Geometry: final body of the model. Coordinates: model frame, mm. Face numbers are marked on the shaded views. A direction names the side the tool comes from. Give positions to 0.01 mm unless a question says otherwise; leave off trailing zeros. Loops run counter-clockwise (first coordinate to the right, second up) from the corner with the lowest first, then second, coordinate; pieces in that order, holes last.
Autodesk Inventor part; units mm, degrees
ref_plane "YZ Plane" through (0, 0, 0) normal (1, 0, 0) x (0, 1, 0)
ref_plane "XZ Plane" through (0, 0, 0) normal (0, 1, 0) x (-1, 0, 0)
ref_plane "XY Plane" through (0, 0, 0) normal (0, 0, 1) x (1, 0, 0)
sketch "Sketch1" plane through (0, 0, 0) normal (0, 0, 1) x (1, 0, 0)
  line L0 (-24.5, 22.5) -> (24.5, 22.5)
  line L1 (29.5, 17.5) -> (29.5, -17.5)
  line L2 (24.5, -22.5) -> (-24.5, -22.5)
  line L3 (-29.5, -17.5) -> (-29.5, 17.5)
  arc A0 (-24.5, 22.5) -> (-29.5, 17.5) centre (-24.5, 17.5) ccw
  arc A1 (29.5, 17.5) -> (24.5, 22.5) centre (24.5, 17.5) ccw
  arc A2 (24.5, -22.5) -> (29.5, -17.5) centre (24.5, -17.5) ccw
  arc A3 (-29.5, -17.5) -> (-24.5, -22.5) centre (-24.5, -17.5) ccw
  line L4 (-24.5, 19.5) -> (24.5, 19.5)
  line L5 (24.5, -19.5) -> (-24.5, -19.5)
  arc A4 (-24.5, 19.5) -> (-26.5, 17.5) centre (-24.5, 17.5) ccw
  arc A5 (-26.5, -17.5) -> (-24.5, -19.5) centre (-24.5, -17.5) ccw
  arc A6 (26.5, 17.5) -> (24.5, 19.5) centre (24.5, 17.5) ccw
  arc A7 (24.5, -19.5) -> (26.5, -17.5) centre (24.5, -17.5) ccw
  line L6 (-26.5, -16.5) -> (-24.5, -16.5)
  line L7 (-24.5, -16.5) -> (-24.5, -14.5)
  line L8 (-24.5, -14.5) -> (-26.5, -14.5)
  line L9 (-26.5, -12.5) -> (-24.5, -12.5)
  line L10 (-24.5, -12.5) -> (-24.5, -10.5)
  line L11 (-24.5, -10.5) -> (-26.5, -10.5)
  line L12 (26.5, -16.5) -> (24.5, -16.5)
  line L13 (24.5, -14.5) -> (26.5, -14.5)
  line L14 (26.5, -12.5) -> (24.5, -12.5)
  line L15 (24.5, -10.5) -> (26.5, -10.5)
  line L16 (-26.5, -10.5) -> (-26.5, 17.5)
  line L17 (-26.5, -17.5) -> (-26.5, -16.5)
  line L18 (-26.5, -14.5) -> (-26.5, -12.5)
  line L19 (26.5, 17.5) -> (26.5, -10.5)
  line L20 (26.5, -12.5) -> (26.5, -14.5)
  line L21 (26.5, -16.5) -> (26.5, -17.5)
  line L22 (24.5, -12.5) -> (24.5, -10.5)
  line L23 (24.5, -16.5) -> (24.5, -14.5)
  point P0 (0, 0)
  point P1 (0, 22.5)
  point P2 (-29.5, 0)
  point P3 (0, 19.5)
  point P4 (-26.5, 0)
  dimension "d0" = 5
  dimension "d1" = 59
  dimension "d2" = 45
  dimension "d4" = 3
  dimension "d6" = 3
  dimension "d7" = 2
  dimension "d8" = 2
  dimension "d9" = 3
extrude "Extrusion1" add sketch "Sketch1" along normal blind 10
sketch "Sketch3" plane through (-29.5, -17.5, 0) normal (-1, 0, 0) x (0, 0, 1)
  line L0 (0, 0) -> (0, 35)
  line L1 (0, 0) -> (10, 0)
  line L2 (10, 35) -> (10, 0)
  line L3 (0, 35) -> (10, 35)
  line L4 (5, 31) -> (5, 4) construction
  point P0 (0, 17.5)
  point P1 (5, 35)
  point P2 (0, 17.5)
  point P3 (5, 17.5)
  dimension "d20" = 27
sketch "Sketch2" plane through (-24.5, 22.5, 0) normal (0, 1, 0) x (1, 0, 0)
  line L0 (0, 0) -> (49, 0)
  line L1 (0, 0) -> (0, -10)
  line L2 (49, -10) -> (0, -10)
  line L3 (49, 0) -> (49, -10)
  line L4 (7, -5) -> (42, -5) construction
  point P0 (24.5, 0)
  point P1 (0, -5)
  point P2 (24.5, 0)
  point P3 (24.5, -5)
  dimension "d12" = 35
hole "Hole1" at (-17.5, 22.5, 5) at (17.5, 22.5, 5) direction (0, -1, 0) diameter 2 end through all
hole "Hole2" at (-29.5, 13.5, 5) at (-29.5, -13.5, 5) direction (1, 0, 0) diameter 2 end through all
equation "\"d4\" = d3"
equation "\"d6\" = d3"
properties part number "Board_holder"
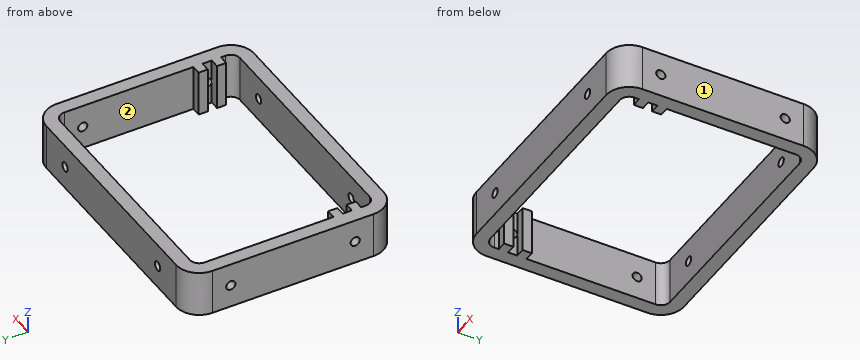
Item 1: Pin query (flat end, axial travel): pin 1 (2.5 mm diameter, centred on x = 17.5, z = 5, fed in from -Y); pin 2 (1.6 mm diameter, centred on x = -25.5, z = 4, fed in from +Y). Return the tip coordinate at first contact, or that it passes through.
Values follow:
pin 1: stops at y = -22.5
pin 2: stops at y = 22.5
Item 2: Ray query, probe 1 along Z at (x, y) = (17.5, 21.3); probe 2 along X at (y, z) = (10, 9.75); probe 3 along Y at (x, z) = (19.5, 2.5). Return the intervals inside material, ascending.
Values follow:
probe 1: z = 0 to 4, 6 to 10
probe 2: x = -29.5 to -26.5, 26.5 to 29.5
probe 3: y = -22.5 to -19.5, 19.5 to 22.5
Item 3: Section query B-B on x = 17.5. Return loops of the section in (y, z), plus the area to 3 significant figures.
Values follow:
outline: (-22.5, 0) - (-19.5, 0) - (-19.5, 4) - (-22.5, 4) - close; (-22.5, 6) - (-19.5, 6) - (-19.5, 10) - (-22.5, 10) - close; (19.5, 0) - (22.5, 0) - (22.5, 4) - (19.5, 4) - close; (19.5, 6) - (22.5, 6) - (22.5, 10) - (19.5, 10) - close
area: 48.0 mm2
Item 4: Section query A-A on y = 5.5. Return loops of the section in (x, z), plus the area to 3 significant figures.
Values follow:
outline: (-29.5, 0) - (-26.5, 0) - (-26.5, 10) - (-29.5, 10) - close; (26.5, 0) - (29.5, 0) - (29.5, 10) - (26.5, 10) - close
area: 60.0 mm2
Item 5: Set-up query: the marked faces 1 and 2. Return all of +Z, -Z, +X, -X, +Y, -Y with unobstructed straight access to the full face (end or side cutting, diameter ignored); none if empty.
Values follow:
face 1: +Z, -Z, +X, +Y, -Y
face 2: +Z, -Z
Item 6: Section query C-C on x = -1.5. Return loops of the section in (y, z), plus the area to 3 significant figures.
Values follow:
outline: (-22.5, 0) - (-19.5, 0) - (-19.5, 10) - (-22.5, 10) - close; (19.5, 0) - (22.5, 0) - (22.5, 10) - (19.5, 10) - close
area: 60.0 mm2
Item 7: Section query D-D on y = 13.5. Return loops of the section in (x, z).
Values follow:
outline: (-29.5, 0) - (-26.5, 0) - (-26.5, 4) - (-29.5, 4) - close; (-29.5, 6) - (-26.5, 6) - (-26.5, 10) - (-29.5, 10) - close; (26.5, 0) - (29.5, 0) - (29.5, 4) - (26.5, 4) - close; (26.5, 6) - (29.5, 6) - (29.5, 10) - (26.5, 10) - close
